from build123d import *

# Parameters (mm, degrees)
F0_R      = 15.94
F1_DEPTH  = 5.34
F1_FACE_R = 15.94
F3_R      = 7.95
F5_DEPTH  = 27
F7_W      = 15.9
F7_H      = 15.9
F8_DEPTH  = 13.7
F10_R     = 5.5
F11_DEPTH = 45
F13_R     = 5.975
F14_DEPTH = 2.5
F16_R     = 3.8
F18_R     = 3.2
F21_R     = 2.05
F22_DEPTH = 175
F23_R     = 3
F24_R     = 1
F26_R     = 13
F27_DEPTH = 3
F28_R     = 2.99999


# Not quite as in the source:
# - a fillet or chamfer is up to 0.001 mm smaller than in the source, because OpenCascade refuses the exact size


with BuildPart() as f1:
    # F0 (on Top) → F1 (new body)
    with BuildSketch(Plane.XY):
        Circle(F0_R)
    extrude(amount=F1_DEPTH)

    # F1_face (on face) → F4 section 0
    with BuildSketch(Plane.XY.offset(5.34)):
        Circle(F1_FACE_R)
    # F3 (on offset) → F4 section 1
    with BuildSketch(Plane.XY.offset(11.18)):
        Circle(F3_R)
    loft()

    # F5 (add): a face of the model
    f5_faces = [f1.faces().sort_by_distance(p)[0] for p in [
        (0, 0, 11.18),
    ]]
    extrude(f5_faces, amount=F5_DEPTH)

    # F7 (on offset) → F8 (join)
    with BuildSketch(Plane.XY.offset(38.18)):
        Rectangle(F7_W, F7_H)
    extrude(amount=F8_DEPTH)

    # F10 (on offset) → F11 (join)
    with BuildSketch(Plane(origin=(0, 7.95, 0), x_dir=(-1, 0, 0), z_dir=(0, 1, 0))):
        with Locations((0, 45.03)):
            Circle(F10_R)
    extrude(amount=F11_DEPTH)

    # F13 (on offset) → F14 (join)
    with BuildSketch(Plane.XY.offset(51.88)):
        Circle(F13_R)
    extrude(amount=F14_DEPTH)

    # F16 (on offset) → F19 section 0
    with BuildSketch(Plane.XY.offset(54.38)):
        Circle(F16_R)
    # F18 (on offset) → F19 section 1
    with BuildSketch(Plane.XY.offset(58.97)):
        Circle(F18_R)
    loft()

    # F21 (on offset) → F22 (join)
    with BuildSketch(Plane.XY.offset(58.97)):
        Circle(F21_R)
    extrude(amount=F22_DEPTH)

    # F23
    f23_edges = [f1.edges().sort_by_distance(p)[0] for p in [
        (-7.95, -7.95, 45.03),
        (-7.95, 7.95, 45.03),
        (7.95, -7.95, 45.03),
        (7.95, 7.95, 45.03),
    ]]
    fillet(f23_edges, radius=F23_R)

    # F24
    f24_edges = [f1.edges().sort_by_distance(p)[0] for p in [
        (-15.94, 0, 0),
    ]]
    fillet(f24_edges, radius=F24_R)

    # F26 (on offset) → F27 (cut)
    with BuildSketch(Plane(origin=(0, 0, 0), x_dir=(1, 0, 0), z_dir=(0, 0, -1))):
        Circle(F26_R)
    extrude(amount=-F27_DEPTH, mode=Mode.SUBTRACT)

    # F28 (radius 3 in the source; OpenCascade refuses exactly that, so slightly less here)
    f28_edges = [f1.edges().sort_by_distance(p)[0] for p in [
        (-13, 0, 3),
    ]]
    fillet(f28_edges, radius=F28_R)


with BuildPart() as f29_1:
    # F29: copy of F1
    add(f1.part)


solid = f1.part
Source: CAD feature listing. Evaluate the final solid. Frame: model axes, mm. A direction names the side the tool comes from. Give positions to 0.01 mm unless a question says otherwise; leave off trailing zeros. Order: outer loops, then holes, each group sorted by start corner. A loop starts at its lowest first (then second) coordinate and runs counter-clockwise, first axis right, second up. Notation, with made-up numbers: (-16.5, -21.75) -> (37.5, -21.75) arc R19 cw to (37.5, -14.75) -> close; hole circle Ø4 at (13, 14). An arc over 180 degrees is marked (long way). Use a Markdown table: item, result.
1) Mould query, pull axis X, two halves, no side actions, for faces 4 (the cylindrical face through (1.19, 30.14, 39.66)), 5 (the flat face through (0, 0, 3)), 6 (the flat face through (-6, -6, 38.18)). Classes: +X half, -X half, draft (parallel to the pull), parting line (faces both ways), or undercut.
Answer list:
| item | result |
|---|---|
| face 4 | parting line |
| face 5 | undercut |
| face 6 | draft |
2) Section query B-B, the plane y = 47.5. Return the cut outline in (x, z), then the cut area to 3 significant figures.
Answer list:
| item | result |
|---|---|
| outline | circle Ø11 at (0, 45.03) |
| area | 95.0 mm² |
3) Section query A-A, the plane z = 33. Return the cut outline in (x, y).
Answer list:
| item | result |
|---|---|
| outline | circle Ø15.9 at (0, 0) |
4) Reachability of faces 1 (the cylindrical face through (3.21, 5.04, 53.11)), 2 (the flat face through (6, -6, 38.18)), 3 (the flat face through (0, 7.95, 51)) from +Z, -Z, +X, -X, +Y, -Y: full face, straight path, thin tool, end or side. Return the list, or none.
Answer list:
| item | result |
|---|---|
| face 1 | +Z |
| face 2 | +X, -Y |
| face 3 | +Z, +Y |
5) Contact query for flat-ended pins moving along their axis: P1, Ø6.5, axis at x = -5, y = -5, coming from the -Z side; P2, Ø5, axis at y = -2.5, z = 46, coming from the -X side; P3, Ø11, axis at y = 2.5, z = 42, coming from the +X side. Output: stop coordinate, or through.
Answer list:
| item | result |
|---|---|
| P1 | z = 2.98 |
| P2 | x = -7.95 |
| P3 | x = 7.95 |
6) Ray query, line 1 along Z through (x, y) = (0, -2.5); line 2 along Z through (x, y) = (-1, 14.5); line 3 along X through (y, z) = (-4.5, 45.5). Return the intervals inside material, ascending. Write a range as [from, to].
Answer list:
| item | result |
|---|---|
| line 1 | [3, 58.97] |
| line 2 | [0, 6.37], [39.62, 50.44] |
| line 3 | [-7.95, 7.95] |
